Autodesk Inventor part; units mm, degrees
ref_plane "GRIFF_XY" through (0, 0, 0) normal (0, 0, -1) x (1, 0, 0)
ref_plane "GRIFF_YZ" through (0, 0, 0) normal (1, 0, 0) x (0, -1, 0)
ref_plane "GRIFF_ZX" through (0, 0, 0) normal (0, -1, 0) x (0, 0, -1)
sketch "Sketch_1" plane through (0, 0, 0) normal (0, 0, 1) x (1, 0, 0)
  line L0 (-5, 10.05) -> (-3, 10.05)
  line L1 (-3, 10.05) -> (-3, 6.5)
  line L2 (-3, 6.5) -> (-5, 6.5)
  line L3 (-5, 6.5) -> (-5, 0)
  line L4 (-5, 0) -> (5, 0)
  line L5 (5, 0) -> (5, 6.5)
  line L6 (5, 6.5) -> (3, 6.5)
  line L7 (3, 6.5) -> (3, 10.05)
  line L8 (3, 10.05) -> (5, 10.05)
  line L9 (5, 10.05) -> (5, 32.5)
  line L10 (5, 32.5) -> (-5, 32.5)
  line L11 (-5, 32.5) -> (-5, 10.05)
extrude "Extrusion1" add sketch "Sketch_1" along normal blind 21.9
sketch "Sketch_2" plane through (0, 0, 0) normal (1, 0, 0) x (0, 1, 0)
  arc A0 (12.5, 8.9) -> (11.5, 7.9) centre (12.5, 7.9) ccw
  line L0 (11.5, 7.9) -> (11.5, 0)
  line L1 (11.5, 0) -> (32.5, 0)
  line L2 (32.5, 0) -> (32.5, 8.9)
  line L3 (32.5, 8.9) -> (12.5, 8.9)
extrude "Extrusion2" cut sketch "Sketch_2" along normal mid plane 10
sketch "Sketch_5" plane through (0, 0, 0) normal (1, 0, 0) x (0, 1, 0)
  line L0 (22.5, 8.9) -> (22.5, 21.9)
  line L1 (22.5, 21.9) -> (24.2, 21.9)
  line L2 (24.2, 21.9) -> (24, 21.7)
  line L3 (24, 21.7) -> (24, 9.1)
  line L4 (24, 9.1) -> (24.2, 8.9)
  line L5 (24.2, 8.9) -> (22.5, 8.9)
  line L6 (22.5, 8.9) -> (22.5, 21.9)
revolve "Revolution1" cut sketch "Sketch_5" angle 360 about axis through (0, 22.5, 8.9) along (0, 0, -1)
sketch "Sketch_6" plane through (0, 0, 0) normal (1, 0, 0) x (0, 1, 0)
  line L0 (17, 8.9) -> (17, 21.9)
  line L1 (17, 21.9) -> (20.7, 21.9)
  line L2 (20.7, 21.9) -> (20.5, 21.7)
  line L3 (20.5, 21.7) -> (20.5, 20.3)
  line L4 (20.5, 20.3) -> (18.621, 20.3)
  line L5 (18.621, 20.3) -> (18.621, 8.9)
  line L6 (18.621, 8.9) -> (17, 8.9)
  line L7 (17, 8.9) -> (17, 21.9)
revolve "Revolution2" cut sketch "Sketch_6" angle 360 about axis through (0, 17, 8.9) along (0, 0, -1)
thread "Thread1"
sketch "Sketch_7" plane through (0, 0, 0) normal (1, 0, 0) x (0, 1, 0)
  line L0 (28, 8.9) -> (28, 21.9)
  line L1 (28, 21.9) -> (31.7, 21.9)
  line L2 (31.7, 21.9) -> (31.5, 21.7)
  line L3 (31.5, 21.7) -> (31.5, 20.3)
  line L4 (31.5, 20.3) -> (29.621, 20.3)
  line L5 (29.621, 20.3) -> (29.621, 8.9)
  line L6 (29.621, 8.9) -> (28, 8.9)
  line L7 (28, 8.9) -> (28, 21.9)
revolve "Revolution3" cut sketch "Sketch_7" angle 360 about axis through (0, 28, 8.9) along (0, 0, -1)
thread "Thread2"
sketch "Sketch_10" plane through (0, 0, 0) normal (0, 1, 0) x (-1, 0, 0)
  line L0 (0.75, 3) -> (-0.75, 3)
  line L1 (-0.75, 3) -> (-0.75, 1.5)
  line L2 (-0.75, 1.5) -> (0.75, 1.5)
  line L3 (0.75, 1.5) -> (0.75, 3)
extrude "Extrusion3" add sketch "Sketch_10" against normal blind 1.5
ref_plane "GRIFF_XY" through (0, 0, 0) normal (0, 0, -1) x (1, 0, 0)
ref_plane "GRIFF_YZ" through (0, 0, 0) normal (1, 0, 0) x (0, -1, 0)
ref_plane "GRIFF_ZX" through (0, 0, 0) normal (0, -1, 0) x (0, 0, -1)
ref_plane "TO_ZBH_1_XY" through (0, 17, 20.3) normal (0, 0, -1) x (1, 0, 0)
ref_plane "TO_ZBH_1_YZ" through (0, 17, 20.3) normal (1, 0, 0) x (0, -1, 0)
ref_plane "TO_ZBH_1_ZX" through (0, 17, 20.3) normal (0, -1, 0) x (0, 0, -1)
ref_plane "TO_ZBH_2_XY" through (0, 28, 20.3) normal (0, 0, -1) x (1, 0, 0)
ref_plane "TO_ZBH_2_YZ" through (0, 28, 20.3) normal (1, 0, 0) x (0, -1, 0)
ref_plane "TO_ZBH_2_ZX" through (0, 28, 20.3) normal (0, -1, 0) x (0, 0, -1)
properties part number "1254044 DHPS-16-A-NO---(Handle)"
The model under review builds one solid part; all positions refer to its coordinate system, in mm. A direction names the side the tool comes from. Give positions to 0.01 mm unless a question says otherwise; leave off trailing zeros. Loops run counter-clockwise (first coordinate to the right, second up) from the corner with the lowest first, then second, coordinate; pieces in that order, holes last. Notation, with made-up numbers: (36.25, -31.75) -> (82.25, -31.75) arc R33 cw to (82.25, 6.25) -> close; hole circle Ø5 at (9, -19.5). An arc over 180 degrees is marked (long way). Answer as a JSON object with one key per item and string values. Group by question number.
Q1. Insertion check: pin 1 (1 mm diameter, centred on x = -3.5, z = 7, fed in from +Y); pin 2 (3.5 mm diameter, centred on x = 0, y = 28, fed in from -Z); pin 3 (3.5 mm diameter, centred on x = -1.5, y = 18, fed in from +Z). Each pin has a flat end and moves straight along its axis. Give the tip position at first contact, or say it passes through.
Q2. Take a section at C-C (z = 7.5). Write out the cut boundary in (x, y), plus the area to 3 significant figures.
Q3. Draft analysis for pull direction X (two halves, no side actions). For faces 6 (the flat face through (0.75, -1, 2)), 7 (the flat face through (-3, 8, 11)), 8 (the flat face through (0, -1, 1.5)), 9 (the cylindrical face through (1.05, 31.34, 20.99)), state which applies: pulls with the +X half, pulls with the -X half, needs draft (parallel to the pull), parting line crosses it, or undercut.
Q4. Tool access review of faces 1 (the flat face through (-2, 29, 20.3)), 2 (the flat face through (4, 10.05, 11)), 3 (the flat face through (0, 25, 8.9)), 4 (the flat face through (-4, 10.05, 11)), 5 (the flat face through (-5, 21, 16)): name each direction out of +Z, -Z, +X, -X, +Y, -Y from which nothing blocks a thin tool from reaching the whole face with its end or side.
Q5. Take a section at B-B (z = 19). Write out the cut boundary in (x, y).
Q6. Take a section at D-D (y = 22.5). Write out the cut boundary in (x, z).
Q7. Wall thickness on line 1 along X through (y, z) = (17, 12.5); line 2 along Y through (x, z) = (3.25, 14.25); line 3 along Y through (x, z) = (-1.25, 16): over which ranges is each line inside the solid? List them lowest first.
Q8. Take a section at A-A (y = 17). Write out the cut boundary in (x, z), plus the area to 3 significant figures.
Answer below:
{
 "1": {"pin 1": "stops at y = 11.5", "pin 2": "stops at z = 8.9", "pin 3": "stops at z = 21.75"},
 "2": {"outline": "(-5, 0) -> (5, 0) -> (5, 6.5) -> (3, 6.5) -> (3, 10.05) -> (5, 10.05) -> (5, 11.5) -> (-5, 11.5) -> (-5, 10.05) -> (-3, 10.05) -> (-3, 6.5) -> (-5, 6.5) -> close", "area": "101 mm2"},
 "3": {"face 6": "pulls with the +X half", "face 7": "pulls with the -X half", "face 8": "needs draft", "face 9": "undercut"},
 "4": {"face 1": "+Z", "face 2": "+Z, -Z, +X", "face 3": "-Z, +X, -X, +Y", "face 4": "+Z, -Z, -X", "face 5": "+Z, -Z, -X, +Y, -Y"},
 "5": {"outline": "(-5, 0) -> (5, 0) -> (5, 6.5) -> (3, 6.5) -> (3, 10.05) -> (5, 10.05) -> (5, 32.5) -> (-5, 32.5) -> (-5, 10.05) -> (-3, 10.05) -> (-3, 6.5) -> (-5, 6.5) -> close; hole circle Ø3.24 at (0, 17); hole circle Ø3.24 at (0, 28); hole circle Ø3 at (0, 22.5)"},
 "6": {"outline": "(-5, 8.9) -> (-1.7, 8.9) -> (-1.5, 9.1) -> (-1.5, 21.7) -> (-1.7, 21.9) -> (-5, 21.9) -> close; (1.5, 9.1) -> (1.7, 8.9) -> (5, 8.9) -> (5, 21.9) -> (1.7, 21.9) -> (1.5, 21.7) -> close"},
 "7": {"line 1": "x = -5 to -1.62, 1.62 to 5", "line 2": "y = 0 to 6.5, 10.05 to 32.5", "line 3": "y = 0 to 15.97, 18.03 to 21.67, 23.33 to 26.97, 29.03 to 32.5"},
 "8": {"outline": "(-5, 8.9) -> (-1.62, 8.9) -> (-1.62, 20.3) -> (-3.5, 20.3) -> (-3.5, 21.7) -> (-3.7, 21.9) -> (-5, 21.9) -> close; (1.62, 8.9) -> (5, 8.9) -> (5, 21.9) -> (3.7, 21.9) -> (3.5, 21.7) -> (3.5, 20.3) -> (1.62, 20.3) -> close", "area": "81.8 mm2"}
}
